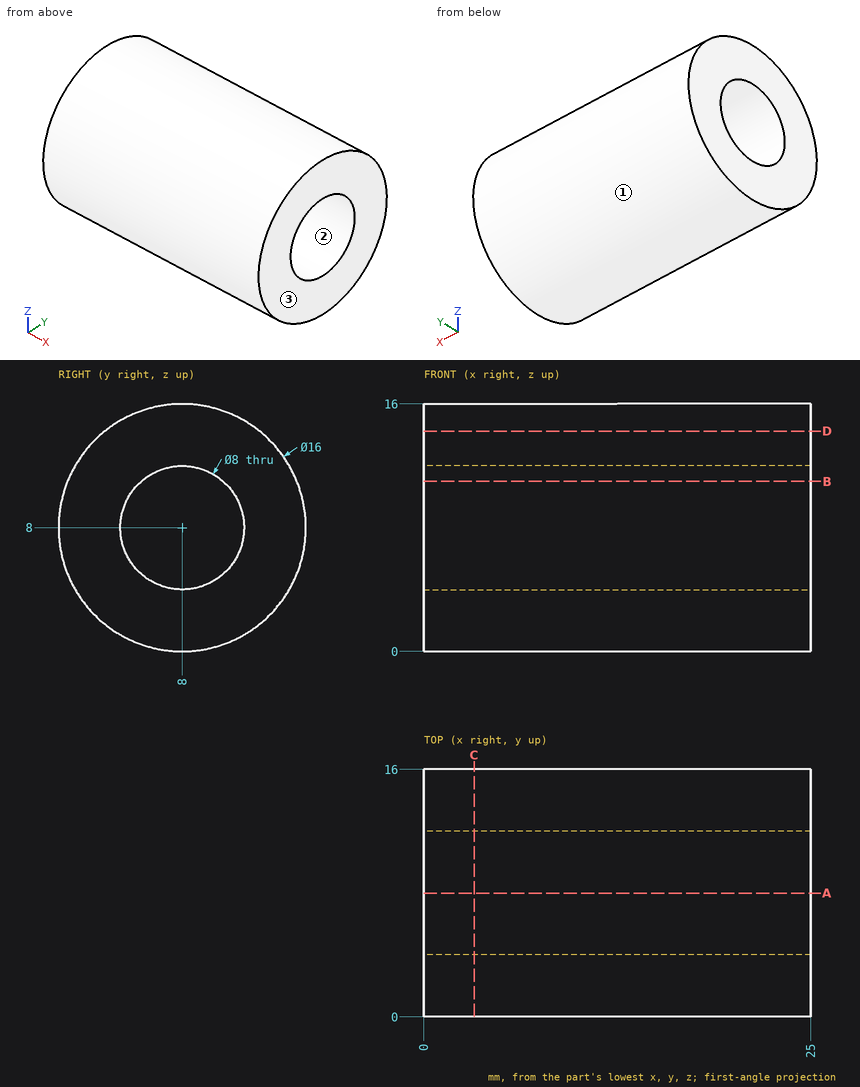
For this review, use the dimensioned drawing (mm, ordinates from the lowest corner) and the shaded views. Give positions to 0.01 mm unless a question says otherwise; leave off trailing zeros. Loops run counter-clockwise (first coordinate to the right, second up) from the corner with the lowest first, then second, coordinate; pieces in that order, holes last.
Item 1: Draft analysis for pull direction Y (two halves, no side actions). For the marked faces 1, 2 and 3, state which applies: +Y half, -Y half, draft (parallel to the pull), parting line (faces both ways), or undercut.
Item 2: Take a section at A-A, the plane y = 8. State the section outline as (x, z) points.
Item 3: Take a section at C-C, the plane x = 3.25. State the section outline as (y, z) points.
Item 4: Take a section at B-B, the plane z = 11. State the section outline as (x, y) points.
Item 5: Take a section at D-D, the plane z = 14.25. State the section outline as (x, y) points, and give its area (3 significant figures).
Item 6: Insertion check: pin 1 (1.5 mm diameter, centred on x = 11, z = 5, fed in from +Y); pin 2 (4 mm diameter, centred on x = 18.5, y = 11.5, fed in from -Z); pin 3 (6.5 mm diameter, centred on y = 8, z = 8, fed in from -X); pin 4 (5 mm diameter, centred on x = 17, z = 12, fed in from +Y). Each pin has a flat end and moves straight along its axis. Give the tip position at first contact, or say it passes through.
Item 7: For line 1 along Y through (x, z) = (7.5, 8); line 2 along Z through (x, y) = (23, 7.5); line 3 along Z through (x, y) = (17.75, 2.5), list the stretches that pass through material, from the lowest coordinate up.
Calculated:
1. face 1: parting line
1. face 2: undercut
1. face 3: draft
2. outline: (0, 0) - (25, 0) - (25, 4) - (0, 4) - close; (0, 12) - (25, 12) - (25, 16) - (0, 16) - close
3. outline: circle Ø16 at (8, 8); hole circle Ø8 at (8, 8)
4. outline: (0, 0.58) - (25, 0.58) - (25, 5.35) - (0, 5.35) - close; (0, 10.65) - (25, 10.65) - (25, 15.42) - (0, 15.42) - close
5. outline: (0, 3.01) - (25, 3.01) - (25, 12.99) - (0, 12.99) - close
5. area: 250 mm2
6. pin 1: stops at y = 15.68
6. pin 2: stops at z = 0.14
6. pin 3: passes through
6. pin 4: stops at y = 15.86
7. line 1: y = 0 to 4, 12 to 16
7. line 2: z = 0.02 to 4.03, 11.97 to 15.98
7. line 3: z = 2.19 to 13.81
